```python
from build123d import *

# Parameters (mm, degrees)
SKETCH1_W                = 3.5
SKETCH1_H                = 16
SKETCH1_W_2              = 21
SKETCH1_H_2              = 6
BOSS_EXTRUDE1_DEPTH      = 10
SKETCH2_R                = 6.5
BOSS_EXTRUDE2_DEPTH      = 6
CUT_EXTRUDE2_DEPTH       = 6
SKETCH5_R                = 1.5
CUT_EXTRUDE3_DEPTH       = 41.10610926
BOSS_EXTRUDE3_DEPTH      = 1.75
BOSS_EXTRUDE3_DEPTH_BACK = 1.75
SKETCH6_R                = 2.277777778
CUT_EXTRUDE6_DEPTH       = 39.967935537
CUT_EXTRUDE6_DEPTH_BACK  = 39.967935537
FILLET1_R                = 1
FILLET2_R                = 5
SKETCH11_R               = 2
CUT_EXTRUDE7_DEPTH       = 41.10610926
SKETCH12_R               = 3
CUT_EXTRUDE8_DEPTH       = 45.371780878
CUT_EXTRUDE9_DEPTH       = 39.967935618
CUT_EXTRUDE9_DEPTH_BACK  = 39.967935618
SKETCH13_R               = 1.5


with BuildPart() as part:
    # Sketch1 → Boss-Extrude1 (new body)
    with BuildSketch(Plane.XY):
        with Locations((1.75, 8)):
            Rectangle(SKETCH1_W, SKETCH1_H)
        with Locations((14, 19)):
            Rectangle(SKETCH1_W_2, SKETCH1_H_2)
        with Locations((1.75, 19)):
            Rectangle(SKETCH1_W, SKETCH1_H_2)
        with Locations((26.25, 19)):
            Rectangle(SKETCH1_W, SKETCH1_H_2)
        with BuildLine():
            Line((28, 16), (24.5, 16))
            Line((24.5, 16), (24.5, 0.5))
            ThreePointArc((24.5, 0.5), (25.525126266, 2.974873734), (28, 4))
            Line((28, 4), (28, 16))
        make_face()
        with BuildLine():
            ThreePointArc((28, 4), (25.525126266, 2.974873734), (24.5, 0.5))
            ThreePointArc((24.5, 0.5), (25.525126266, -1.974873734), (28, -3))
            Line((28, -3), (28, 4))
        make_face()
        with BuildLine():
            ThreePointArc((31.5, 0.5), (30.474873734, 2.974873734), (28, 4))
            Line((28, 4), (28, -3))
            ThreePointArc((28, -3), (30.474873734, -1.974873734), (31.5, 0.5))
        make_face()
        with BuildLine():
            ThreePointArc((28, 4), (25.525126266, 2.974873734), (24.5, 0.5))
            ThreePointArc((24.5, 0.5), (25.525126266, -1.974873734), (28, -3))
            Line((28, -3), (28, 4))
        make_face()
        with BuildLine():
            ThreePointArc((31.5, 0.5), (30.474873734, 2.974873734), (28, 4))
            Line((28, 4), (28, -3))
            ThreePointArc((28, -3), (30.474873734, -1.974873734), (31.5, 0.5))
        make_face()
    extrude(amount=BOSS_EXTRUDE1_DEPTH)

    # Sketch2 → Boss-Extrude2 (add)
    with BuildSketch(Plane(origin=(0, 22, 0), x_dir=(1, 0, 0), z_dir=(0, 1, 0))):
        with Locations((14, -5)):
            Circle(SKETCH2_R)
    extrude(amount=-BOSS_EXTRUDE2_DEPTH)

    # Sketch4 → Cut-Extrude2 (cut)
    with BuildSketch(Plane(origin=(0, 22, 0), x_dir=(1, 0, 0), z_dir=(0, 1, 0))):
        with BuildLine():
            Line((17.122498999, -2.5), (10.877501001, -2.5))
            ThreePointArc((10.877501001, -2.5), (10, -5), (10.877501001, -7.5))
            Line((10.877501001, -7.5), (17.122498999, -7.5))
            ThreePointArc((17.122498999, -7.5), (17.774254628, -6.324764885), (18, -5))
            ThreePointArc((18, -5), (17.774254628, -3.675235115), (17.122498999, -2.5))
        make_face()
        with BuildLine():
            Line((20, -2.5), (17.122498999, -2.5))
            ThreePointArc((17.122498999, -2.5), (17.774254628, -3.675235115), (18, -5))
            ThreePointArc((18, -5), (17.774254628, -6.324764885), (17.122498999, -7.5))
            Line((17.122498999, -7.5), (20, -7.5))
            Line((20, -7.5), (20, -2.5))
        make_face()
        with BuildLine():
            Line((10.877501001, -2.5), (8, -2.5))
            Line((8, -2.5), (8, -7.5))
            Line((8, -7.5), (10.877501001, -7.5))
            ThreePointArc((10.877501001, -7.5), (10, -5), (10.877501001, -2.5))
        make_face()
        with BuildLine():
            ThreePointArc((17.122498999, -2.5), (14, -1), (10.877501001, -2.5))
            Line((10.877501001, -2.5), (17.122498999, -2.5))
        make_face()
        with BuildLine():
            Line((17.122498999, -7.5), (10.877501001, -7.5))
            ThreePointArc((10.877501001, -7.5), (14, -9), (17.122498999, -7.5))
        make_face()
    extrude(amount=-CUT_EXTRUDE2_DEPTH, mode=Mode.SUBTRACT)

    # Sketch5 → Cut-Extrude3 (cut, through all)
    with BuildSketch(Plane.XY.offset(10)):
        with Locations((28, 0.5)):
            Circle(SKETCH5_R)
    extrude(amount=-CUT_EXTRUDE3_DEPTH, mode=Mode.SUBTRACT)

    # Sketch6 → Boss-Extrude3 (add, two sides: drawn at the far end of the back side and taken through both)
    with BuildSketch(Plane.XY.offset(5).offset(-BOSS_EXTRUDE3_DEPTH_BACK)):
        with BuildLine():
            Line((0, 9), (0, 19))
            Line((0, 19), (-7.866666667, 13.1))
            ThreePointArc((-7.866666667, 13.1), (-5.48134681, 13.315084157), (-4.222222222, 11.277777778))
            ThreePointArc((-4.222222222, 11.277777778), (-4.889367887, 9.667145665), (-6.5, 9))
            Line((-6.5, 9), (0, 9))
        make_face()
        with Locations((-6.5, 11.277777778)):
            Circle(SKETCH6_R)
    extrude(amount=BOSS_EXTRUDE3_DEPTH + BOSS_EXTRUDE3_DEPTH_BACK)

    # Sketch10 → Cut-Extrude6 (cut, two sides: drawn at the far end of the back side and taken through both)
    with BuildSketch(Plane.XY.offset(5).offset(-CUT_EXTRUDE6_DEPTH_BACK)):
        Polygon((0, 22), (0, 19), (2.784123139, 21.274018631), (3.672955578, 22), align=None)
    extrude(amount=CUT_EXTRUDE6_DEPTH + CUT_EXTRUDE6_DEPTH_BACK, mode=Mode.SUBTRACT)

    # Fillet1
    fillet1_edges = [part.edges().sort_by_distance(p)[0] for p in [
        (28, 22, 5),
    ]]
    fillet(fillet1_edges, radius=FILLET1_R)

    # Fillet2
    fillet2_edges = [part.edges().sort_by_distance(p)[0] for p in [
        (1.75, 0, 0),
        (1.75, 0, 10),
    ]]
    fillet(fillet2_edges, radius=FILLET2_R - 0.0001)  # a hair under: the kernel refuses the full size

    # Sketch11 → Cut-Extrude7 (cut, through all)
    with BuildSketch(Plane(origin=(0, 0, 0), x_dir=(0, 0, -1), z_dir=(1, 0, 0))):
        with Locations(Location((-5, 6, 0), (0, 0, 270))):
            Circle(SKETCH11_R)
    extrude(amount=CUT_EXTRUDE7_DEPTH, mode=Mode.SUBTRACT)

    # Sketch12 → Cut-Extrude8 (cut, through all)
    with BuildSketch(Plane(origin=(28, 0, 0), x_dir=(0, 0, -1), z_dir=(1, 0, 0))):
        with Locations((-5, 6)):
            Circle(SKETCH12_R)
    extrude(amount=CUT_EXTRUDE8_DEPTH, mode=Mode.SUBTRACT)

    # Sketch13 → Cut-Extrude9 (cut, two sides: drawn at the far end of the back side and taken through both)
    with BuildSketch(Plane.XY.offset(5).offset(-CUT_EXTRUDE9_DEPTH_BACK)):
        with Locations((-6.5, 11.277777778)):
            Circle(SKETCH13_R)
    extrude(amount=CUT_EXTRUDE9_DEPTH + CUT_EXTRUDE9_DEPTH_BACK, mode=Mode.SUBTRACT)


solid = part.part
```
Here's how the part is built. I have some questions about the finished solid (model axes, mm). A direction names the side the tool comes from. Coordinates: 2 decimals unless noted, no trailing zeros. Loops run counter-clockwise (first coordinate to the right, second up) from the corner with the lowest first, then second, coordinate; pieces in that order, holes last. Notation, with made-up numbers: (87, 44) - (105, 44) arc R30 cw to (105, 83) - close; hole circle Ø5 at (19.5, -8.75). An arc over 180 degrees is marked (long way). Return JSON: item names as keys, results as strings. Group by question number.
Item 1: We'd pull the mould along Z, two halves only. Please class faces 6 (the face through (13.9, 19, 11.5)), 7 (the face through (19, 19, 7.5)), 8 (the face through (27.699, 21.715, 5.07)): +Z half, -Z half, draft (parallel to the pull), parting line (faces both ways), or undercut.
Item 2: I need wall thicknesses on line 1 (X direction, y = 9.75, z = 1); line 2 (Z direction, x = 1.5, y = 6); line 3 (Z direction, x = 9, y = 17.5). Which ranges of each line are inside material? Lowest first, please. Write a range as from..to.
Item 3: On a 3-axis mill with a long thin cutter (end or side, diameter ignored), from which of +Z, -Z, +X, -X, +Y, -Y can I reach the whole of each face in a straight line? I mean faces 1 (the face through (29, 3, 5)), 2 (the face through (2, 2, 1)), 3 (the face through (2, 2, 9)), 4 (the face through (3.5, 10, 5)), 5 (the face through (8, 19, 5)). Say none if no direction works.
Item 4: If we section it at B-B on y = 6: Write out the boundary of the cut face in (x, z), and give its area (3 significant figures).
Item 5: If we section it at C-C on x = 14.5: Write out the boundary of the cut face in (y, z).
Item 6: If we section it at A-A on z = 8: Write out the boundary of the cut face in (x, y), and give its area (3 significant figures).
Item 7: Will these pins go through, and if not, where does the flat tip stop? P1, Ø1.4, axis at x = 10, y = 18.5, coming from the +Z side; P2, Ø4, axis at x = 27.5, y = 7, coming from the -Z side; P3, Ø3.5, axis at y = 6, z = 5, coming from the +X side; P4, Ø3, axis at y = 10.5, z = 4.5, coming from the +X side.
Item 8: If we section it at D-D on y = 20.25: Write out the boundary of the cut face in (x, z), and give its area (3 significant figures).
Calculated:
{
 "1": {"face 6": "+Z half", "face 7": "undercut", "face 8": "draft"},
 "2": {"line 1": "x = 0..3.5, 24.5..28", "line 2": "z = 0..3, 7..10", "line 3": "z = 0..2.5, 7.5..10"},
 "3": {"face 1": "+X, +Y", "face 2": "-Z, -X, -Y", "face 3": "+Z, -X, -Y", "face 4": "+Z, -Z, -Y", "face 5": "+Y, -Y"},
 "4": {"outline": "(0, 0) - (3.5, 0) - (3.5, 3) - (0, 3) - close; (0, 7) - (3.5, 7) - (3.5, 10) - (0, 10) - close; (24.5, 0) - (28, 0) - (28, 3) - (24.5, 3) - close; (24.5, 7) - (28, 7) - (28, 10) - (24.5, 10) - close", "area": "42.0 mm^2"},
 "5": {"outline": "(16, -1.48) - (22, -1.48) - (22, 1.03) - (16, 1.03) - close; (16, 8.97) - (22, 8.97) - (22, 11.48) - (16, 11.48) - close"},
 "6": {"outline": "(0, 1) - (3.5, 1) - (3.5, 16) - (11.35, 16) - (11.35, 22) - (3.67, 22) - (0, 19) - close; (16.65, 16) - (24.5, 16) - (24.5, 0.5) arc R3.5 ccw (long way) to (28, 4) - (28, 21) arc R1 ccw to (27, 22) - (16.65, 22) - close; hole circle Ø3 at (28, 0.5)", "area": "259 mm^2"},
 "7": {"P1": "stops at z = 10.6", "P2": "stops at z = 0", "P3": "passes through", "P4": "stops at x = 28"},
 "8": {"outline": "(1.53, 0) - (9.85, 0) arc R6.5 ccw to (18.15, 0) - (28, 0) - (28, 10) - (18.15, 10) arc R6.5 ccw to (9.85, 10) - (1.53, 10) - close; hole (8, 2.5) - (10.88, 2.5) arc R4 ccw to (17.12, 2.5) - (20, 2.5) - (20, 7.5) - (17.12, 7.5) arc R4 ccw to (10.88, 7.5) - (8, 7.5) - close", "area": "209 mm^2"}
}
